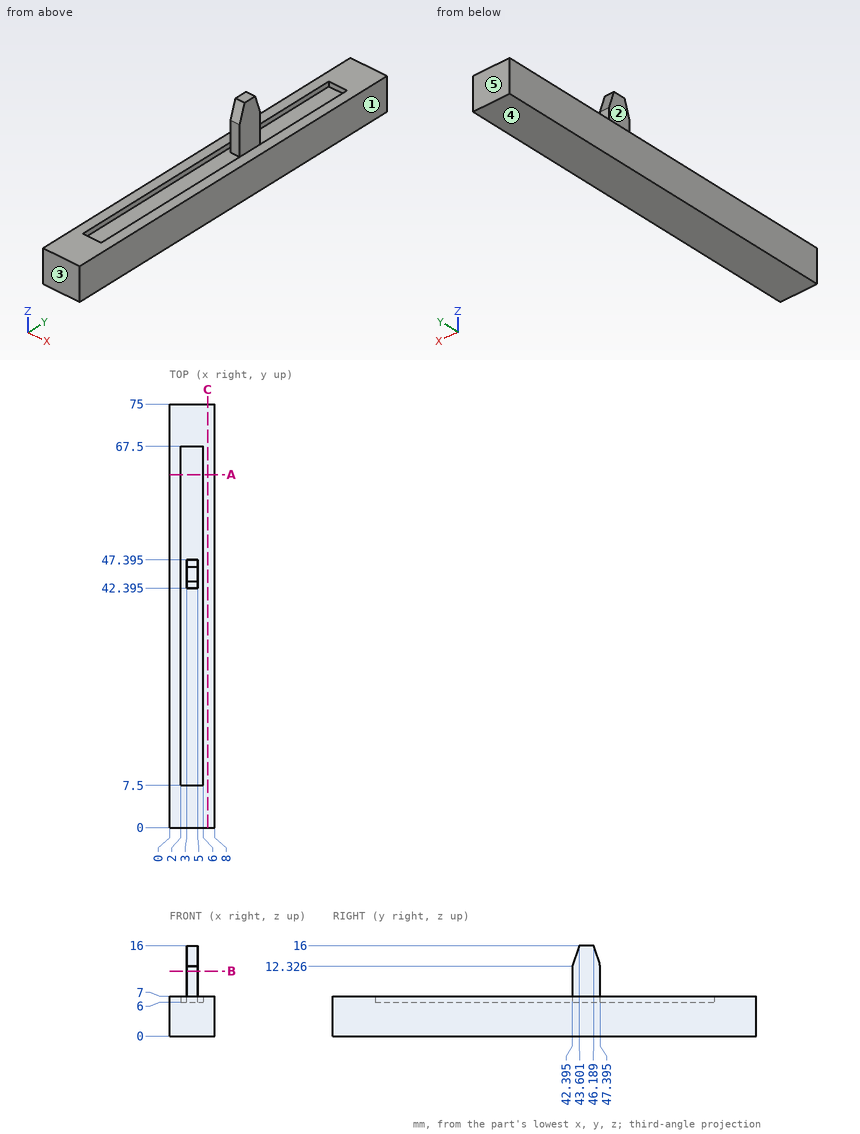
Check sheet for the drawn part. Datum: minimum x, y, z corner. Units: mm. A direction names the side the tool comes from. Coordinates: 2 decimals unless noted, no trailing zeros. Write each loop counter-clockwise with the first axis right and the second up, starting at its lowest first coordinate (ties: lowest second). Pieces come first, ordered by that corner, then holes. Notation, with made-up numbers: (29.25, -18) - (36.25, -18) arc R22 ccw to (36.25, 19) - close; hole circle Ø3 at (8, 5.25). An arc over 180 degrees is marked (long way). Answer as a JSON object with one key per item and string values.
(1) Gauge pin test, flat ends, axial feed: pin 1 Ø4 at (x, y) = (5.5, 28.5) entering from +Z; pin 2 Ø3 at (x, z) = (3.5, 11.5) entering from +Y (1 decimal); pin 3 Ø2 at (x, y) = (4, 37.5) entering from +Z; pin 4 Ø8 at (y, z) = (65, 13.5) entering from +X. Record the tip position at first contact, or that the pin passes through.
Report:
{"pin 1": "z = 7", "pin 2": "y = 47.4", "pin 3": "z = 6", "pin 4": "through"}
(2) Cross-section at A-A on y = 62.5. Record the cut outline in (x, z).
Report:
{"outline": "(0, 0) - (8, 0) - (8, 7) - (6, 7) - (6, 6) - (2, 6) - (2, 7) - (0, 7) - close"}
(3) Thickness scan on line 1 along Y through (x, z) = (4, 6.5) (1 decimal); line 2 along Z through (x, y) = (7, 27.5); line 3 along Z through (x, y) = (2.5, 13). Record the ranges inside material, lowest first.
Report:
{"line 1": "0 to 7.5, 42.4 to 47.4, 67.5 to 75", "line 2": "0 to 7", "line 3": "0 to 6"}
(4) Mould release check, pull along Y, two halves, no side actions. Record for the marked faces 3, 4 and 5: pulls with the +Y half, pulls with the -Y half, needs draft (parallel to the pull), parting line crosses it, or undercut.
Report:
{"face 3": "pulls with the -Y half", "face 4": "needs draft", "face 5": "pulls with the +Y half"}
(5) Cross-section at B-B on z = 11.5. Record the cut outline in (x, y) (1 decimal).
Report:
{"outline": "(3, 42.4) - (5, 42.4) - (5, 47.4) - (3, 47.4) - close"}
(6) Tool access check on the marked faces 1 and 2. Record the directions out of +Z, -Z, +X, -X, +Y, -Y that give a thin tool (end or side, any length) a straight path to the whole face; none if there is none.
Report:
{"face 1": "+Z, -Z, +X, +Y, -Y", "face 2": "+Z"}
(7) Cross-section at C-C on x = 6.75. Record the cut outline in (y, z), plus the area to 3 significant figures.
Report:
{"outline": "(0, 0) - (75, 0) - (75, 7) - (0, 7) - close", "area": "525 mm^2"}
